from build123d import *

# Parameters (mm, degrees)
SKETCH1_W                = 100
SKETCH1_H                = 90
SKETCH1_W_2              = 90
SKETCH1_H_2              = 80
BOSS_EXTRUDE1_DEPTH      = 70
SKETCH2_W                = 100
SKETCH2_H                = 90
BOSS_EXTRUDE2_DEPTH      = 5
FILLET1_R                = 5
SKETCH3_R                = 1.55
CUT_EXTRUDE1_DEPTH       = 146.430395722
SKETCH4_R                = 3
CUT_EXTRUDE2_DEPTH       = 2.5
CUT_EXTRUDE3_DEPTH       = 146.430395722
SKETCH6_W                = 12.5
SKETCH6_H                = 5
REVOLVE2_ANGLE           = 90
SKETCH7_W                = 12.5
SKETCH7_H                = 5
REVOLVE3_ANGLE           = 90
SKETCH8_W                = 12.5
SKETCH8_H                = 5
REVOLVE4_ANGLE           = 90
SKETCH9_W                = 12.5
SKETCH9_H                = 5
REVOLVE5_ANGLE           = 90
SKETCH10_R               = 1.55
CUT_EXTRUDE5_DEPTH       = 5
SKETCH13_R               = 3.75
BOSS_EXTRUDE3_DEPTH      = 5
SKETCH14_R               = 1.55
CUT_EXTRUDE7_DEPTH       = 146.430395722
FILLET3_R                = 5
CUT_EXTRUDE8_DEPTH       = 5
FILLET4_R                = 2.5
CUT_EXTRUDE11_DEPTH      = 149.744747806
CUT_EXTRUDE11_DEPTH_BACK = 149.744747806


with BuildPart() as part:
    # Sketch1 → Boss-Extrude1 (new body)
    with BuildSketch(Plane(origin=(0, 0, 0), x_dir=(1, 0, 0), z_dir=(0, 1, 0))):
        with Locations((45, 40)):
            Rectangle(SKETCH1_W, SKETCH1_H)
        with Locations((45, 40)):
            Rectangle(SKETCH1_W_2, SKETCH1_H_2, mode=Mode.SUBTRACT)
    extrude(amount=BOSS_EXTRUDE1_DEPTH)

    # Sketch2 → Boss-Extrude2 (add)
    with BuildSketch(Plane(origin=(0, 0, 0), x_dir=(-1, 0, 0), z_dir=(0, -1, 0))):
        with Locations((-45, 40)):
            Rectangle(SKETCH2_W, SKETCH2_H)
    extrude(amount=BOSS_EXTRUDE2_DEPTH)

    # Fillet1
    fillet1_edges = [part.edges().sort_by_distance(p)[0] for p in [
        (-5, 32.5, -85),
        (95, 32.5, -85),
        (95, 32.5, 5),
        (-5, 32.5, 5),
    ]]
    fillet(fillet1_edges, radius=FILLET1_R)

    # Sketch3 → Cut-Extrude1 (cut, through all)
    with BuildSketch(Plane(origin=(0, 0, 0), x_dir=(1, 0, 0), z_dir=(0, 1, 0))):
        with Locations(Location((16.5, 68.5, 0), (0, 0, 270))):
            Circle(SKETCH3_R)
        with Locations(Location((16.5, 11.5, 0), (0, 0, 270))):
            Circle(SKETCH3_R)
        with Locations(Location((73.5, 11.5, 0), (0, 0, 270))):
            Circle(SKETCH3_R)
        with Locations(Location((73.5, 68.5, 0), (0, 0, 270))):
            Circle(SKETCH3_R)
    extrude(amount=-CUT_EXTRUDE1_DEPTH, mode=Mode.SUBTRACT)

    # Sketch4 → Cut-Extrude2 (cut)
    with BuildSketch(Plane(origin=(0, -5, 0), x_dir=(-1, 0, 0), z_dir=(0, -1, 0))):
        with Locations(Location((-16.5, 11.5, 0), (0, 0, 90))):
            Circle(SKETCH4_R)
        with Locations(Location((-73.5, 11.5, 0), (0, 0, 90))):
            Circle(SKETCH4_R)
        with Locations(Location((-73.5, 68.5, 0), (0, 0, 90))):
            Circle(SKETCH4_R)
        with Locations(Location((-16.5, 68.5, 0), (0, 0, 90))):
            Circle(SKETCH4_R)
    extrude(amount=-CUT_EXTRUDE2_DEPTH, mode=Mode.SUBTRACT)

    # Sketch5 → Cut-Extrude3 (cut, through all)
    with BuildSketch(Plane(origin=(0, 0, 0), x_dir=(1, 0, 0), z_dir=(0, 1, 0))):
        with BuildLine():
            Line((26, 65), (26, 15))
            ThreePointArc((26, 15), (25, 14), (24, 15))
            Line((24, 15), (24, 65))
            ThreePointArc((24, 65), (25, 66), (26, 65))
        make_face()
        with BuildLine():
            Line((66, 65), (66, 15))
            ThreePointArc((66, 15), (65, 14), (64, 15))
            Line((64, 15), (64, 65))
            ThreePointArc((64, 65), (65, 66), (66, 65))
        make_face()
        with BuildLine():
            Line((52.666666667, 65), (52.666666667, 15))
            ThreePointArc((52.666666667, 15), (51.666666667, 14), (50.666666667, 15))
            Line((50.666666667, 15), (50.666666667, 65))
            ThreePointArc((50.666666667, 65), (51.666666667, 66), (52.666666667, 65))
        make_face()
        with BuildLine():
            Line((39.333333333, 65), (39.333333333, 15))
            ThreePointArc((39.333333333, 15), (38.333333333, 14), (37.333333333, 15))
            Line((37.333333333, 15), (37.333333333, 65))
            ThreePointArc((37.333333333, 65), (38.333333333, 66), (39.333333333, 65))
        make_face()
    extrude(amount=-CUT_EXTRUDE3_DEPTH, mode=Mode.SUBTRACT)

    # Sketch6 → Revolve2 (revolve)
    with BuildSketch(Plane.XY.offset(-80)):
        with Locations((6.25, 67.5)):
            Rectangle(SKETCH6_W, SKETCH6_H)
    revolve(axis=Axis((0, 70, -80), (0, -1, 0)), revolution_arc=REVOLVE2_ANGLE)

    # Sketch7 → Revolve3 (revolve)
    with BuildSketch(Plane.XY.offset(-80)):
        with Locations((83.75, 67.5)):
            Rectangle(SKETCH7_W, SKETCH7_H)
    revolve(axis=Axis((90, 70, -80), (0, 1, 0)), revolution_arc=REVOLVE3_ANGLE)

    # Sketch8 → Revolve4 (revolve)
    with BuildSketch(Plane(origin=(0, 0, 0), x_dir=(-1, 0, 0), z_dir=(0, 0, -1))):
        with Locations((-83.75, 67.5)):
            Rectangle(SKETCH8_W, SKETCH8_H)
    revolve(axis=Axis((90, 70, 0), (0, -1, 0)), revolution_arc=REVOLVE4_ANGLE)

    # Sketch9 → Revolve5 (revolve)
    with BuildSketch(Plane(origin=(0, 0, 0), x_dir=(-1, 0, 0), z_dir=(0, 0, -1))):
        with Locations((-6.25, 67.5)):
            Rectangle(SKETCH9_W, SKETCH9_H)
    revolve(axis=Axis((0, 70, 0), (0, 1, 0)), revolution_arc=REVOLVE5_ANGLE)

    # Sketch10 → Cut-Extrude5 (cut)
    with BuildSketch(Plane(origin=(0, 70, 0), x_dir=(1, 0, 0), z_dir=(0, 1, 0))):
        with Locations(Location((5, 75, 0), (0, 0, 270))):
            Circle(SKETCH10_R)
        with Locations(Location((85, 75, 0), (0, 0, 270))):
            Circle(SKETCH10_R)
        with Locations(Location((85, 5, 0), (0, 0, 270))):
            Circle(SKETCH10_R)
        with Locations(Location((5, 5, 0), (0, 0, 270))):
            Circle(SKETCH10_R)
    extrude(amount=-CUT_EXTRUDE5_DEPTH, mode=Mode.SUBTRACT)

    # Sketch13 → Boss-Extrude3 (add)
    with BuildSketch(Plane(origin=(0, 0, 0), x_dir=(1, 0, 0), z_dir=(0, 1, 0))):
        with Locations(Location((16.5, 68.5, 0), (0, 0, 90))):
            Circle(SKETCH13_R)
        with Locations(Location((73.5, 68.5, 0), (0, 0, 90))):
            Circle(SKETCH13_R)
        with Locations(Location((73.5, 11.5, 0), (0, 0, 90))):
            Circle(SKETCH13_R)
        with Locations(Location((16.5, 11.5, 0), (0, 0, 90))):
            Circle(SKETCH13_R)
    extrude(amount=BOSS_EXTRUDE3_DEPTH)

    # Sketch14 → Cut-Extrude7 (cut, through all)
    with BuildSketch(Plane(origin=(0, 0, 0), x_dir=(-1, 0, 0), z_dir=(0, -1, 0))):
        with Locations(Location((-73.5, 68.5, 0), (0, 0, 270))):
            Circle(SKETCH14_R)
        with Locations(Location((-73.5, 11.5, 0), (0, 0, 270))):
            Circle(SKETCH14_R)
        with Locations(Location((-16.5, 11.5, 0), (0, 0, 270))):
            Circle(SKETCH14_R)
        with Locations(Location((-16.5, 68.5, 0), (0, 0, 270))):
            Circle(SKETCH14_R)
    extrude(amount=-CUT_EXTRUDE7_DEPTH, mode=Mode.SUBTRACT)

    # Fillet3
    fillet3_edges = [part.edges().sort_by_distance(p)[0] for p in [
        (-5, -5, -40),
        (45, -5, -85),
        (95, -5, -40),
        (45, -5, 5),
        (-3.535533906, -5, 3.535533906),
        (93.535533906, -5, 3.535533906),
        (93.535533906, -5, -83.535533906),
        (-3.535533906, -5, -83.535533906),
    ]]
    fillet(fillet3_edges, radius=FILLET3_R)

    # Sketch15 → Cut-Extrude8 (cut)
    with BuildSketch(Plane(origin=(0, 0, -85), x_dir=(-1, 0, 0), z_dir=(0, 0, -1))):
        with BuildLine():
            Line((-65, 42.5), (-59.92, 42.5))
            ThreePointArc((-59.92, 42.5), (-52.42, 35), (-59.92, 27.5))
            Line((-59.92, 27.5), (-65, 27.5))
            ThreePointArc((-65, 27.5), (-72.5, 35), (-65, 42.5))
        make_face()
    extrude(amount=-CUT_EXTRUDE8_DEPTH, mode=Mode.SUBTRACT)

    # Fillet4
    fillet4_edges = [part.edges().sort_by_distance(p)[0] for p in [
        (62.46, 42.5, -85),
        (62.46, 27.5, -85),
        (62.46, 42.5, -80),
        (62.46, 27.5, -80),
        (52.42, 35, -85),
        (52.42, 35, -80),
        (72.5, 35, -85),
        (72.5, 35, -80),
    ]]
    fillet(fillet4_edges, radius=FILLET4_R - 0.0001)  # a hair under: the kernel refuses the full size

    # Sketch16 → Cut-Extrude11 (cut, two sides: drawn at the far end of the back side and taken through both)
    with BuildSketch(Plane(origin=(-5, 0, 0), x_dir=(0, 0, -1), z_dir=(1, 0, 0)).offset(-CUT_EXTRUDE11_DEPTH_BACK)):
        with BuildLine():
            Line((65, 55), (65, 15))
            ThreePointArc((65, 15), (64, 14), (63, 15))
            Line((63, 15), (63, 55))
            ThreePointArc((63, 55), (64, 56), (65, 55))
        make_face()
        with BuildLine():
            Line((47, 15), (47, 55))
            ThreePointArc((47, 55), (48, 56), (49, 55))
            Line((49, 55), (49, 15))
            ThreePointArc((49, 15), (48, 14), (47, 15))
        make_face()
        with BuildLine():
            Line((17, 55), (17, 15))
            ThreePointArc((17, 15), (16, 14), (15, 15))
            Line((15, 15), (15, 55))
            ThreePointArc((15, 55), (16, 56), (17, 55))
        make_face()
        with BuildLine():
            Line((33, 55), (33, 15))
            ThreePointArc((33, 15), (32, 14), (31, 15))
            Line((31, 15), (31, 55))
            ThreePointArc((31, 55), (32, 56), (33, 55))
        make_face()
    extrude(amount=CUT_EXTRUDE11_DEPTH + CUT_EXTRUDE11_DEPTH_BACK, mode=Mode.SUBTRACT)


solid = part.part
The listing builds one solid part. Answer for the finished solid, in the listing's coordinates (mm). A direction names the side the tool comes from. Round coordinates to 2 decimals unless told otherwise and drop trailing zeros. Order: outer loops, then holes, each group sorted by start corner. A loop starts at its lowest first (then second) coordinate and runs counter-clockwise, first axis right, second up. Notation, with made-up numbers: (6, 41) -> (28, 41) arc R24 ccw to (28, 53) -> close; hole circle Ø1 at (31.25, 53). An arc over 180 degrees is marked (long way). Write each question's results on one line, items separated by ' | '. Start each with the question number.
Q1. Each of these flat-tipped pins is pushed along its axis until it touches: pin 1 (2.5 mm diameter, centred on x = 92.5, y = 38.5, fed in from -Z); pin 2 (1.5 mm diameter, centred on x = 92, y = 40.5, fed in from +Z); pin 3 (1.9 mm diameter, centred on x = 85, z = -5, fed in from +Y). Where does it stop, or does it pass through?
Q2. Find section B-B (x = 85). Determine the outline of the cut face in (y, z), then the cut area to 3 significant figures.
Q3. Find section A-A (z = -38.5). Determine the outline of the cut face in (x, y).
Q4. Find section C-C (y = 52). Give the number of separate pieces and of enclosed holes in the cut face, then the cut area to 3 significant figures.
Q5. The mould has two halves that part along X. Classify faces 1 (the flat face through (6.3, 65, -73.7)), 2 (the flat face through (-3, 35, -15)): pulls with the +X half, pulls with the -X half, needs draft (parallel to the pull), parting line crosses it, or undercut.
Q6. Which of the six approach directions +Z, -Z, +X, -X, +Y, -Y give full straight-line access (tool end or side, diameter ignored) to faces 3 (the flat face through (37.333, -2, -40)), 4 (the flat face through (92, 35, -33)), 5 (the cylindrical face through (86.537, 67.535, -5.202))?
Q7. Straight lines are drawn through the part: probe 1 along Z at (x, y) = (73.5, 2.5); probe 2 along X at (y, z) = (20, -10.5); probe 3 along Z at (x, y) = (20, 54). For each, find the intervals that lie inside material, in ascending order. Write a range as from..to.
Worked answers:
1) pin 1: stops at z = -84.84 | pin 2: stops at z = 4.84 | pin 3: stops at y = 0
2) outline: (-5, -80) arc R5 ccw to (0, -85) -> (70, -85) -> (70, -76.55) -> (65, -76.55) -> (65, -80) -> (0, -80) -> (0, 0) -> (65, 0) -> (65, -3.45) -> (70, -3.45) -> (70, 5) -> (0, 5) arc R5 ccw to (-5, 0) -> close; (65, -73.45) -> (70, -73.45) -> (70, -68.54) -> (65, -68.54) -> close; (65, -11.46) -> (70, -11.46) -> (70, -6.55) -> (65, -6.55) -> close | area: 1,220 mm2
3) outline: (-5, 0) arc R5 ccw to (0, -5) -> (24, -5) -> (24, 0) -> (0, 0) -> (0, 70) -> (-5, 70) -> close; (26, -5) -> (37.33, -5) -> (37.33, 0) -> (26, 0) -> close; (39.33, -5) -> (50.67, -5) -> (50.67, 0) -> (39.33, 0) -> close; (52.67, -5) -> (64, -5) -> (64, 0) -> (52.67, 0) -> close; (66, -5) -> (90, -5) arc R5 ccw to (95, 0) -> (95, 70) -> (90, 70) -> (90, 0) -> (66, 0) -> close
4) separate pieces: 8 | enclosed holes: 0 | area: 1,700 mm2
5) face 1: undercut | face 2: needs draft
6) face 3: +Y, -Y | face 4: +X, -X | face 5: +Y
7) probe 1: z = -85..-80, -72.25..-70.05, -66.95..-64.75, -15.25..-13.05, -9.95..-7.75, 0..5 | probe 2: x = -5..0, 90..95 | probe 3: z = -85..-80, 0..5
